```python
from build123d import *

# Parameters (mm, degrees)
SKETCH1_W                    = 19.05
SKETCH1_H                    = 158.75
BOSS_EXTRUDE1_DEPTH          = 6.35
F_1_4_20_TAPPED_HOLE1_D      = 5.1054
F_1_4_0_475_DIAMETER_HOLE1_D = 12.065
CHAMFER1_SIZE                = 6.35


with BuildPart() as part:
    # Sketch1 → Boss-Extrude1 (new body)
    with BuildSketch(Plane.XY):
        with Locations((9.525, 79.375)):
            Rectangle(SKETCH1_W, SKETCH1_H)
    extrude(amount=BOSS_EXTRUDE1_DEPTH)

    # 1/4-20 Tapped Hole1 (through all)
    with Locations(Plane.XY.offset(6.35)):
        with Locations((9.525, 149.225)):
            Hole(F_1_4_20_TAPPED_HOLE1_D / 2)

    # 1/4 (0.475) Diameter Hole1 (through all)
    with Locations(Plane.XY.offset(6.35)):
        with Locations((9.525, 9.525)):
            Hole(F_1_4_0_475_DIAMETER_HOLE1_D / 2)

    # Chamfer1
    chamfer1_edges = [part.edges().sort_by_distance(p)[0] for p in [
        (0, 158.75, 3.175),
        (19.05, 158.75, 3.175),
    ]]
    chamfer(chamfer1_edges, length=CHAMFER1_SIZE)


solid = part.part
```
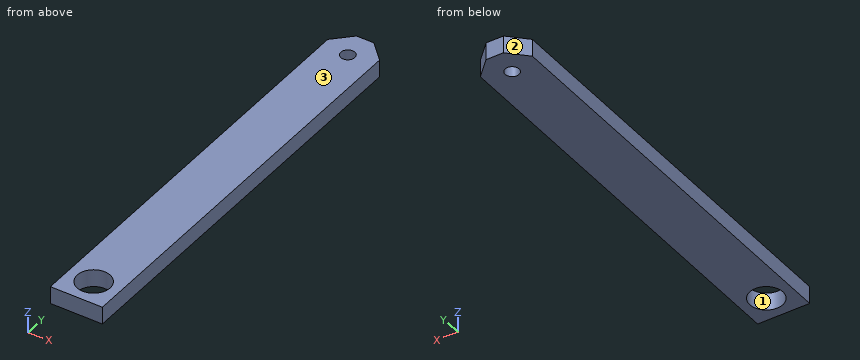
Read the model definition and answer for the solid it produces. Units are mm, in the model's axes. Face numbers are marked on the shaded views. Give positions to 0.01 mm unless a question says otherwise; leave off trailing zeros. Write each loop counter-clockwise with the first axis right and the second up, starting at its lowest first coordinate (ties: lowest second). Pieces come first, ordered by that corner, then holes. Notation, with made-up numbers: (77.25, -21) - (94.25, -21) arc R27 cw to (94.25, 15) - close; hole circle Ø9 at (-3.75, 48.25). An arc over 180 degrees is marked (long way). Write item = value, one per line. Start each with the question number.
Item 1: Each of these flat-tipped pins is pushed along its axis until it touches: P1, Ø3, axis at x = 9.525, y = 149.225, coming from the -Z side; P2, Ø1.5, axis at x = 15.5, z = 3, coming from the +Y side. Where does it stop, or does it pass through?
Item 2: Find section A-A (x = 8.5). Give the vertices of the cut face in (y, z).
Item 3: The mould has two halves that part along Y. Classify the marked faces 1, 2 and 3: +Y half, -Y half, draft (parallel to the pull), parting line (faces both ways), or undercut.
Item 4: Find section B-B (z = 1.25). State how many separate pieces and enclosed holes the cut face has, then the cut area to 3 significant figures.
Item 5: Find the intervals of material crossed by probe 1 along Y at (x, z) = (7.25, 3.5); probe 2 along Y at (x, z) = (9, 5.75); probe 3 along Y at (x, z) = (14, 5.5), in increasing order. Write a range as [from, to].
Item 6: Find section C-C (x = 17.25). Give the vertices of the cut face in (y, z).
Response:
q1.P1 = through
q1.P2 = 156.7
q2.outline = (0, 0) - (3.58, 0) - (3.58, 6.35) - (0, 6.35) - close; (15.47, 0) - (146.89, 0) - (146.89, 6.35) - (15.47, 6.35) - close; (151.56, 0) - (158.75, 0) - (158.75, 6.35) - (151.56, 6.35) - close
q3.face_1 = undercut
q3.face_2 = +Y half
q3.face_3 = draft
q4.separate_pieces = 1
q4.enclosed_holes = 2
q4.area = 2,850 mm²
q5.probe_1 = [0, 3.94], [15.11, 148.07], [150.38, 158.75]
q5.probe_2 = [0, 3.52], [15.53, 146.73], [151.72, 158.75]
q5.probe_3 = [0, 5.48], [13.57, 157.45]
q6.outline = (0, 0) - (154.2, 0) - (154.2, 6.35) - (0, 6.35) - close
